Check sheet for the modelled part. Datum: model origin and axes. Units: mm. Round coordinates to 2 decimals unless told otherwise and drop trailing zeros. Write each loop counter-clockwise with the first axis right and the second up, starting at its lowest first coordinate (ties: lowest second). Pieces come first, ordered by that corner, then holes. Notation, with made-up numbers: (-36.75, 2) - (22.25, 2) arc R15 cw to (22.25, 27) - close; hole circle Ø5 at (76, -34.5). An arc over 180 degrees is marked (long way). Use one line per item in the form item = value. Start each with the question number.
1) Section check B-B (x = -23.5). Record the boundary of the cut face in (y, z), then the cut area to 3 significant figures.
2) Scan lines: probe 1 along X at (y, z) = (56, 2.2); probe 2 along X at (y, z) = (-37, 2.85); probe 3 along Y at (x, z) = (-40, 1.1) (3 decimals). Record each from-to range of solid material in increasing order.
3) Section check C-C (y = -35). Record the boundary of the cut face in (x, z).
4) Section check A-A (y = 55). Record the boundary of the cut face in (x, z).
5) Section check D-D (x = 64). Record the boundary of the cut face in (y, z), then the cut area to 3 significant figures.
6) Gauge pin test, flat ends, axial feed: P1, Ø4, axis at x = -32, y = -10, coming from the -Z side; P2, Ø1.5, axis at y = 40, z = 1.5, coming from the +X side; P3, Ø4.5, axis at x = -55, y = 55, coming from the +Z side. Record the tip position at first contact, or that the pin passes through.
from build123d import *

# Parameters (mm, degrees)
IZIM1_R                     = 100
Y_KSEKLIK_EKSTR_ZYON1_DEPTH = 30
KES_EKSTR_ZYON1_DEPTH       = 145.568322948
M5_BO_LUKLU_DELIK2_D        = 5.5
IZIM20_R                    = 183.537558205
KES_EKSTR_ZYON2_DEPTH       = 27
M4_BO_LUKLU_DELIK1_D        = 4.5
M4_BO_LUKLU_DELIK2_D        = 4.5


with BuildPart() as part:
    # Çizim1 → Yükseklik-Ekstrüzyon1 (new body)
    with BuildSketch(Plane.XY):
        Circle(IZIM1_R)
    extrude(amount=Y_KSEKLIK_EKSTR_ZYON1_DEPTH)

    # Çizim9 → Kes-Ekstrüzyon1 (cut, through all)
    with BuildSketch(Plane.XY.offset(30)):
        with BuildLine():
            Line((27, 65), (27, 25))
            ThreePointArc((27, 25), (23.5, 21.5), (20, 25))
            Line((20, 25), (20, 65))
            ThreePointArc((20, 65), (23.5, 68.5), (27, 65))
        make_face()
        with BuildLine():
            Line((-20, 65), (-20, 25))
            ThreePointArc((-20, 25), (-23.5, 21.5), (-27, 25))
            Line((-27, 25), (-27, 65))
            ThreePointArc((-27, 65), (-23.5, 68.5), (-20, 65))
        make_face()
        with BuildLine():
            Line((-20, -25), (-20, -65))
            ThreePointArc((-20, -65), (-23.5, -68.5), (-27, -65))
            Line((-27, -65), (-27, -25))
            ThreePointArc((-27, -25), (-23.5, -21.5), (-20, -25))
        make_face()
        with BuildLine():
            Line((20, -65), (20, -25))
            ThreePointArc((20, -25), (23.5, -21.5), (27, -25))
            Line((27, -25), (27, -65))
            ThreePointArc((27, -65), (23.5, -68.5), (20, -65))
        make_face()
    extrude(amount=-KES_EKSTR_ZYON1_DEPTH, mode=Mode.SUBTRACT)

    # M5 Boşluklu Delik2 (through all)
    with Locations(Plane.XY.offset(30)):
        with Locations((-55, 55), (55, 55), (55, -55), (-55, -55)):
            Hole(M5_BO_LUKLU_DELIK2_D / 2)

    # Çizim20 → Kes-Ekstrüzyon2 (cut)
    with BuildSketch(Plane.XY.offset(30)):
        with Locations((0, 8.479468632)):
            Circle(IZIM20_R)
    extrude(amount=-KES_EKSTR_ZYON2_DEPTH, mode=Mode.SUBTRACT)

    # M4 Boşluklu Delik1 (through all)
    with Locations(Plane.XY.offset(3)):
        with Locations((-13.265, 40), (-13.265, 70), (13.265, 70), (13.265, 40)):
            Hole(M4_BO_LUKLU_DELIK1_D / 2)

    # M4 Boşluklu Delik2 (through all)
    with Locations(Plane.XY.offset(3)):
        with Locations((40, 13.265), (70, 13.265), (70, -13.265), (40, -13.265), (-40, -12.99677614), (-40, 13.265), (-70, 13.53322386), (-70, -12.99677614), (-13.265, -40), (13.265, -40), (13.265, -70), (-13.265, -70)):
            Hole(M4_BO_LUKLU_DELIK2_D / 2)


solid = part.part
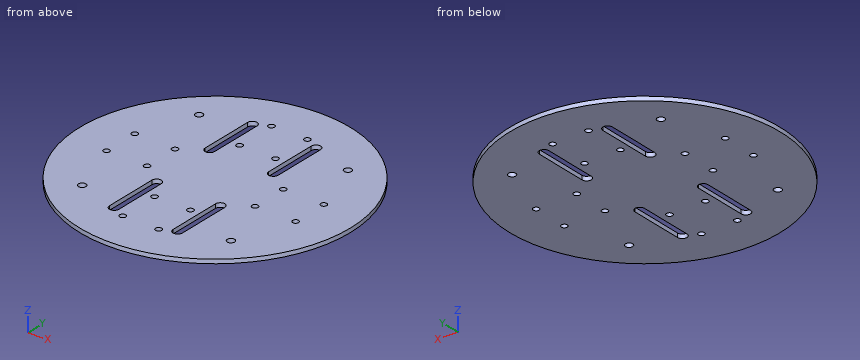
Results are:
q1.outline = (-97.2, 0) - (-68.5, 0) - (-68.5, 3) - (-97.2, 3) - close; (-21.5, 0) - (21.5, 0) - (21.5, 3) - (-21.5, 3) - close; (68.5, 0) - (97.2, 0) - (97.2, 3) - (68.5, 3) - close
q1.area = 301 mm²
q2.probe_1 = -82.85 to -57.56, -52.44 to -27, -20 to 20, 27 to 52.44, 57.56 to 82.85
q2.probe_2 = -92.9 to -27, -20 to 20, 27 to 92.9
q2.probe_3 = -91.652 to -15.247, -10.747 to 11.015, 15.515 to 91.652
q3.outline = (-93.67, 0) - (-27, 0) - (-27, 3) - (-93.67, 3) - close; (-20, 0) - (20, 0) - (20, 3) - (-20, 3) - close; (27, 0) - (93.67, 0) - (93.67, 3) - (27, 3) - close
q4.outline = (-83.52, 0) - (-57.75, 0) - (-57.75, 3) - (-83.52, 3) - close; (-52.25, 0) - (-27, 0) - (-27, 3) - (-52.25, 3) - close; (-20, 0) - (20, 0) - (20, 3) - (-20, 3) - close; (27, 0) - (52.25, 0) - (52.25, 3) - (27, 3) - close; (57.75, 0) - (83.52, 0) - (83.52, 3) - (57.75, 3) - close
q5.outline = (-76.84, 0) - (76.84, 0) - (76.84, 3) - (-76.84, 3) - close
q5.area = 461 mm²
q6.P1 = 0
q6.P2 = 91.98
q6.P3 = through
